```python
from build123d import *

# Parameters (mm, degrees)
MODEL_R                 = 1.5
SALIENTE_EXTRUIR1_DEPTH = 3


with BuildPart() as part:
    # Model → Saliente-Extruir1 (new body)
    with BuildSketch(Plane.XY):
        with BuildLine():
            Line((256.429131311, 228.742243614), (364.429131311, 228.742243614))
            ThreePointArc((364.429131311, 228.742243614), (367.611111826, 227.424224129), (368.929131311, 224.242243614))
            Line((368.929131311, 224.242243614), (368.929131311, 215.242243614))
            ThreePointArc((368.929131311, 215.242243614), (367.611111826, 212.060263099), (364.429131311, 210.742243614))
            Line((364.429131311, 210.742243614), (256.429131311, 210.742243614))
            ThreePointArc((256.429131311, 210.742243614), (253.247150795, 212.060263099), (251.929131311, 215.242243614))
            Line((251.929131311, 215.242243614), (251.929131311, 224.242243614))
            ThreePointArc((251.929131311, 224.242243614), (253.247150795, 227.424224129), (256.429131311, 228.742243614))
        make_face()
        with Locations((310.429131311, 224.242243614)):
            Circle(MODEL_R, mode=Mode.SUBTRACT)
        with Locations((292.429131311, 224.242243614)):
            Circle(MODEL_R, mode=Mode.SUBTRACT)
        with Locations((301.429131311, 224.242243614)):
            Circle(MODEL_R, mode=Mode.SUBTRACT)
        with Locations((337.429131311, 215.242243614)):
            Circle(MODEL_R, mode=Mode.SUBTRACT)
        with Locations((319.429131311, 215.242243614)):
            Circle(MODEL_R, mode=Mode.SUBTRACT)
        with Locations((328.429131311, 215.242243614)):
            Circle(MODEL_R, mode=Mode.SUBTRACT)
        with Locations((310.429131311, 215.242243614)):
            Circle(MODEL_R, mode=Mode.SUBTRACT)
        with Locations((292.429131311, 215.242243614)):
            Circle(MODEL_R, mode=Mode.SUBTRACT)
        with Locations((301.429131311, 215.242243614)):
            Circle(MODEL_R, mode=Mode.SUBTRACT)
        with Locations((274.429131311, 215.242243614)):
            Circle(MODEL_R, mode=Mode.SUBTRACT)
        with Locations((283.429131311, 215.242243614)):
            Circle(MODEL_R, mode=Mode.SUBTRACT)
        with Locations((265.429131311, 215.242243614)):
            Circle(MODEL_R, mode=Mode.SUBTRACT)
        with Locations((256.429131311, 215.242243614)):
            Circle(MODEL_R, mode=Mode.SUBTRACT)
        with Locations((346.429131311, 215.242243614)):
            Circle(MODEL_R, mode=Mode.SUBTRACT)
        with Locations((274.429131311, 224.242243614)):
            Circle(MODEL_R, mode=Mode.SUBTRACT)
        with Locations((265.429131311, 224.242243614)):
            Circle(MODEL_R, mode=Mode.SUBTRACT)
        with Locations((256.429131311, 224.242243614)):
            Circle(MODEL_R, mode=Mode.SUBTRACT)
        with Locations((283.429131311, 224.242243614)):
            Circle(MODEL_R, mode=Mode.SUBTRACT)
        with Locations((337.429131311, 224.242243614)):
            Circle(MODEL_R, mode=Mode.SUBTRACT)
        with Locations((319.429131311, 224.242243614)):
            Circle(MODEL_R, mode=Mode.SUBTRACT)
        with Locations((328.429131311, 224.242243614)):
            Circle(MODEL_R, mode=Mode.SUBTRACT)
        with Locations((346.429131311, 224.242243614)):
            Circle(MODEL_R, mode=Mode.SUBTRACT)
        with Locations((355.429131311, 215.242243614)):
            Circle(MODEL_R, mode=Mode.SUBTRACT)
        with Locations((355.429131311, 224.242243614)):
            Circle(MODEL_R, mode=Mode.SUBTRACT)
        with Locations((364.429131311, 215.242243614)):
            Circle(MODEL_R, mode=Mode.SUBTRACT)
        with Locations((364.429131311, 224.242243614)):
            Circle(MODEL_R, mode=Mode.SUBTRACT)
    extrude(amount=SALIENTE_EXTRUIR1_DEPTH)


solid = part.part
```
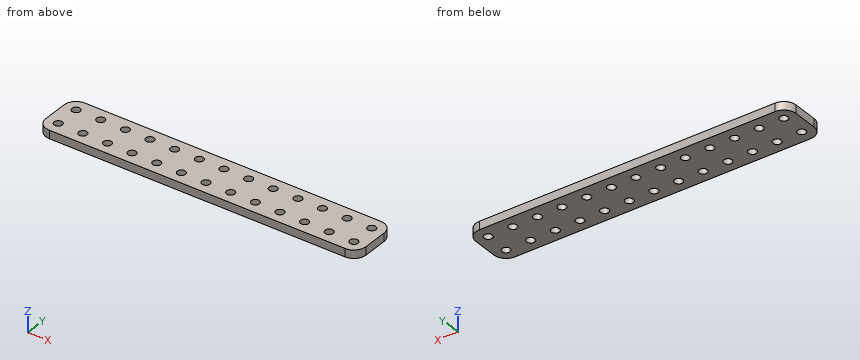
For this review, take the finished solid that the model builds, in its own axes (mm). Round coordinates to 2 decimals unless told otherwise and drop trailing zeros. Write each loop counter-clockwise with the first axis right and the second up, starting at its lowest first coordinate (ties: lowest second). Pieces come first, ordered by that corner, then holes. Notation, with made-up numbers: (34, -7) - (92, -7) arc R20 ccw to (92, 24) - close; hole circle Ø2 at (78.5, -16). An arc over 180 degrees is marked (long way). Answer as a JSON object with one key per item and string values.
1. We need section A-A on z = 1.2. Count the separate pieces of the cut face and the enclosed holes in it, then the cut area to 3 significant figures.
Response values:
{"separate pieces": "1", "enclosed holes": "26", "area": "1,900 mm2"}
2. We need section C-C on y = 227.25. Give the boundary of the cut face in (x, z), then the cut area to 3 significant figures.
Response values:
{"outline": "(253.08, 0) - (367.78, 0) - (367.78, 3) - (253.08, 3) - close", "area": "344 mm2"}
3. We need section B-B on x = 283.5. Give the boundary of the cut face in (y, z).
Response values:
{"outline": "(210.74, 0) - (213.74, 0) - (213.74, 3) - (210.74, 3) - close; (216.74, 0) - (222.74, 0) - (222.74, 3) - (216.74, 3) - close; (225.74, 0) - (228.74, 0) - (228.74, 3) - (225.74, 3) - close"}
4. To check wall thickness, follow line 1 along Y through (x, z) = (329.5, 0.3); line 2 along Y through (x, z) = (311, 2.5); line 3 along X through (y, z) = (226.5, 2.1). State the ranges of each line that lie inside material, in increasing order.
Response values:
{"line 1": "y = 210.74 to 214.19, 216.29 to 223.19, 225.29 to 228.74", "line 2": "y = 210.74 to 213.86, 216.63 to 222.86, 225.63 to 228.74", "line 3": "x = 252.54 to 368.32"}
